```python
from build123d import *

# Parameters (mm, degrees)
F0_W     = 125
F0_H     = 75
F1_DEPTH = 70
F2_W     = 70
F2_H     = 25
F3_DEPTH = 70.001
F5_DEPTH = 75.001


with BuildPart() as f1:
    # F0 (on Front) → F1 (new body)
    with BuildSketch(Plane.XZ):
        with Locations((62.5, 37.5)):
            Rectangle(F0_W, F0_H)
    extrude(amount=-F1_DEPTH)

    # F2 (on face) → F3 (cut, through all)
    with BuildSketch(Plane.XZ):
        with Locations((60, 62.5)):
            Rectangle(F2_W, F2_H)
    extrude(amount=-F3_DEPTH, mode=Mode.SUBTRACT)

    # F4 (on Top) → F5 (cut, through all)
    with BuildSketch(Plane.XY):
        Polygon((105, 0), (105, 30), (70, 30), (70, 35), (40, 35), (40, 20), (0, 20), (0, -31.133723), (125, -31.133723), (125, 0), align=None)
    extrude(amount=F5_DEPTH, mode=Mode.SUBTRACT)


solid = f1.part
```
Build history of the part. All positions in model axes, mm. A direction names the side the tool comes from. Coordinates: 2 decimals unless noted, no trailing zeros. Order: outer loops, then holes, each group sorted by start corner. A loop starts at its lowest first (then second) coordinate and runs counter-clockwise, first axis right, second up.
Item 1: Tool access for faces 5 (the flat face through (113, 35, 75)), 6 (the flat face through (95, 50, 62)), 7 (the flat face through (105, 15, 37)), 8 (the flat face through (20, 20, 37)), 9 (the flat face through (0, 45, 37)): list every direction of +Z, -Z, +X, -X, +Y, -Y with a clear straight run to the whole face (end or side of a thin tool).
Filled in:
face 5: +Z, +X, -X, +Y, -Y
face 6: +Z, +Y, -Y
face 7: +Z, -Z, -Y
face 8: +Z, -Z, -X, -Y
face 9: +Z, -Z, -X, +Y, -Y
Item 2: Drop flat-ended pins along their axis: pin 1 Ø9 at (y, z) = (11, 34) entering from -X; pin 2 Ø20 at (x, z) = (24.5, 43) entering from -Y; pin 3 Ø24 at (x, z) = (60.5, 37) entering from -Y. Give the stop position or say it passes through.
Filled in:
pin 1: stops at x = 105
pin 2: stops at y = 20
pin 3: stops at y = 30
Item 3: Saw through at D-D on x = 27.5. List the corners of the cut face in (y, z), then the cut area to 3 significant figures.
Filled in:
outline: (20, 0) - (70, 0) - (70, 50) - (20, 50) - close
area: 2,500 mm2
Item 4: Drill centre lines: L1, parallel to X at y = 25.5, z = 54; L2, parallel to Y at x = 14, z = 56.5; L3, parallel to Y at x = 102.5, z = 40. Where is each one in solid material? Low to high.
Filled in:
L1: x = 0 to 25, 105 to 125
L2: y = 20 to 70
L3: y = 30 to 70
Item 5: Saw through at A-A on y = 54. List the corners of the cut face in (x, z).
Filled in:
outline: (0, 0) - (125, 0) - (125, 75) - (95, 75) - (95, 50) - (25, 50) - (25, 75) - (0, 75) - close
Item 6: Saw through at C-C on y = 33.5. List the corners of the cut face in (x, z), then the cut area to 4 significant figures.
Filled in:
outline: (0, 0) - (40, 0) - (40, 50) - (25, 50) - (25, 75) - (0, 75) - close; (70, 0) - (125, 0) - (125, 75) - (95, 75) - (95, 50) - (70, 50) - close
area: 6,125 mm2
Item 7: Saw through at B-B on z = 13. List the corners of the cut face in (x, y), then the cut area to 3 significant figures.
Filled in:
outline: (0, 20) - (40, 20) - (40, 35) - (70, 35) - (70, 30) - (105, 30) - (105, 0) - (125, 0) - (125, 70) - (0, 70) - close
area: 5,850 mm2
Item 8: Mould opens along X. For faces 1 (the flat face through (62, 70, 30)), 2 (the flat face through (88, 30, 29)), 3 (the flat face through (40, 28, 25)), 4 (the flat face through (125, 35, 37)) say: released by +X, released by -X, zero draft, split by the parting line, or undercut.
Filled in:
face 1: zero draft
face 2: undercut
face 3: undercut
face 4: released by +X
